Job drawing, mm, ordinate dimensions from the low corner. One solid piece. Round coordinates to 2 decimals unless told otherwise and drop trailing zeros. Loops run counter-clockwise (first coordinate to the right, second up) from the corner with the lowest first, then second, coordinate; pieces in that order, holes last. Notation, with made-up numbers: M 73.5,-34 L 88.5,-34 A12 cw 88.5,-22 Z; hole C -27.75,-35.75 d11. An arc over 180 degrees is marked long. Use one line per item in the form item = value.
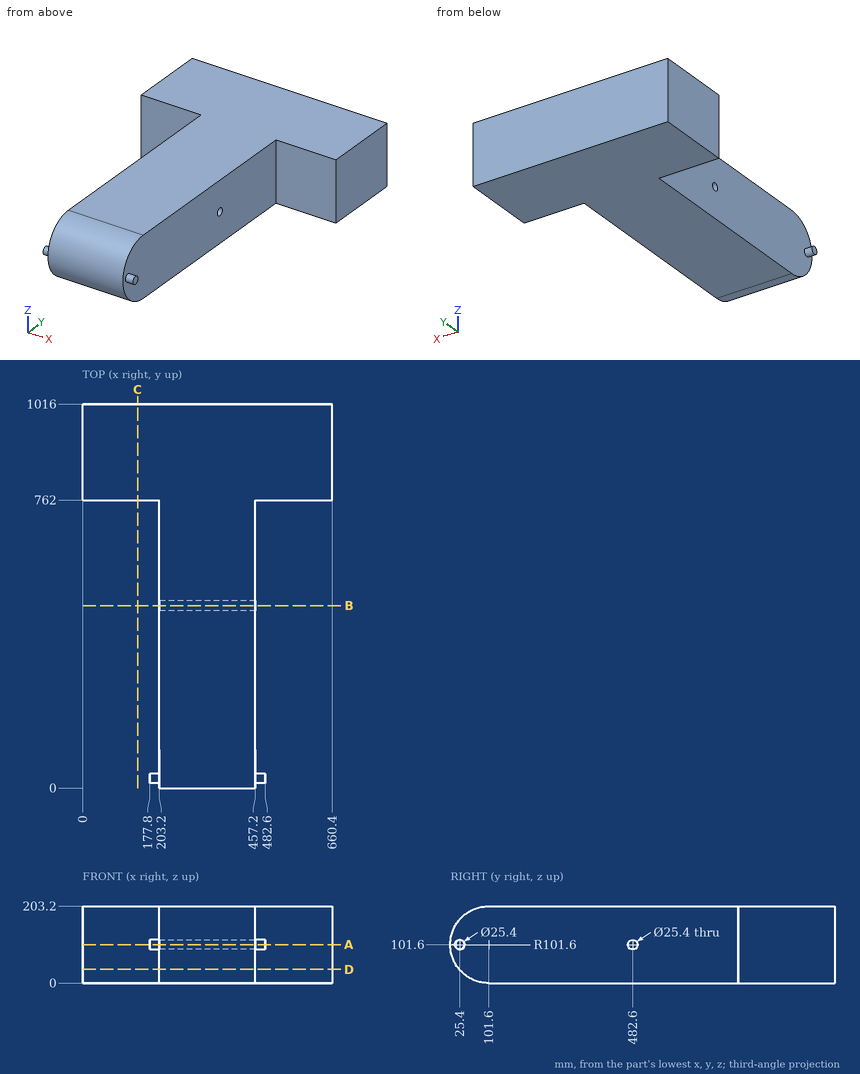
1. Cut at C-C on x = 146. Write the cut outline in (y, z).
Completed:
outline = M 762,0 L 1016,0 L 1016,203.2 L 762,203.2 Z
2. Cut at D-D on z = 36.5. Write the cut outline in (x, y), and give its area (3 significant figures).
Completed:
outline = M 0,762 L 203.2,762 L 203.2,23.6 L 457.2,23.6 L 457.2,762 L 660.4,762 L 660.4,1016 L 0,1016 Z
area = 355,000 mm2
3. Drop flat-ended pins along their axis: P1, Ø1, axis at y = 535.5, z = 61, coming from the -X side; P2, Ø1.5, axis at x = 511, z = 44.5, coming from the -Y side; P3, Ø7.5, axis at y = 30.5, z = 96.5, coming from the -X side. Give the stop position or say it passes through.
Completed:
P1 = 203.2
P2 = 762
P3 = 177.8
4. Cut at B-B on y = 482.6. Write the cut outline in (x, z), and give its area (3 significant figures).
Completed:
outline = M 203.2,0 L 457.2,0 L 457.2,88.9 L 203.2,88.9 Z; M 203.2,114.3 L 457.2,114.3 L 457.2,203.2 L 203.2,203.2 Z
area = 45,200 mm2
5. Probe line 1 along Y through (x, z) = (374, 101.6); line 2 along Z through (x, y) = (276, 482); line 3 along Y through (x, z) = (527, 90). List the from-to ranges inside material, lowest first. Write a range as from..to.
Completed:
line_1 = 0..469.9, 495.3..1016
line_2 = 0..88.91, 114.29..203.2
line_3 = 762..1016
6. Cut at A-A on z = 101.6. Write the cut outline in (x, y).
Completed:
outline = M 0,762 L 203.2,762 L 203.2,495.3 L 457.2,495.3 L 457.2,762 L 660.4,762 L 660.4,1016 L 0,1016 Z; M 177.8,12.7 L 203.2,12.7 L 203.2,0 L 457.2,0 L 457.2,12.7 L 482.6,12.7 L 482.6,38.1 L 457.2,38.1 L 457.2,469.9 L 203.2,469.9 L 203.2,38.1 L 177.8,38.1 Z
